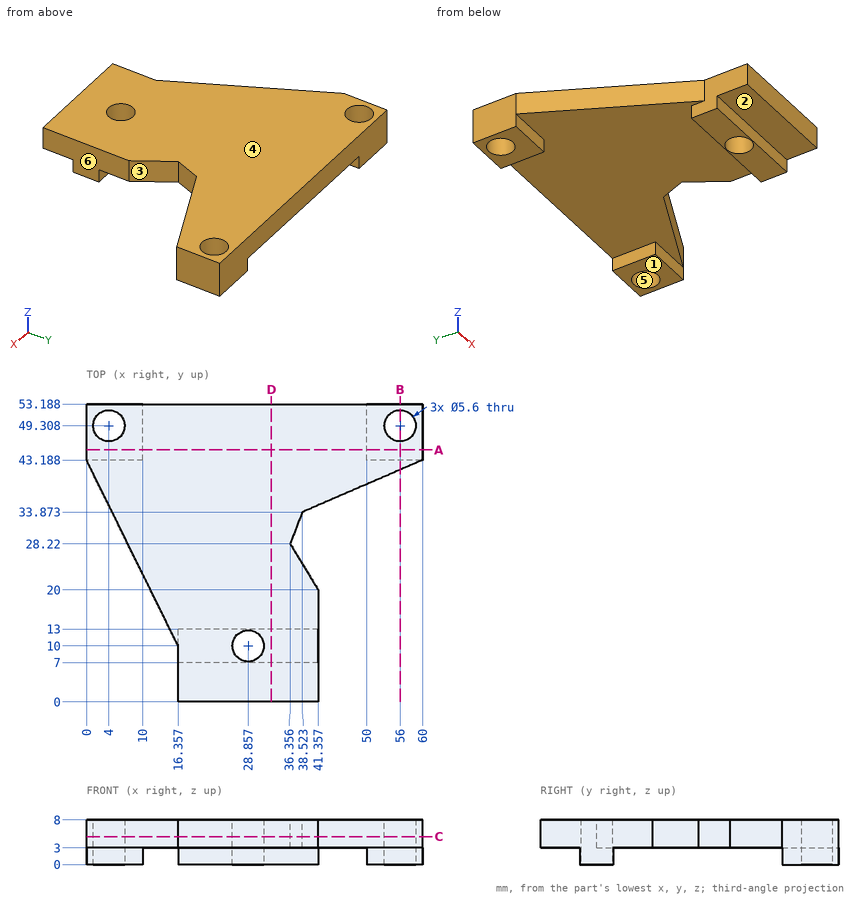
The drawing under review shows one solid part. Ordinate dimensions are in mm from its lowest x, y, z. A direction names the side the tool comes from. Give positions to 0.01 mm unless a question says otherwise; leave off trailing zeros. Order: outer loops, then holes, each group sorted by start corner. A loop starts at its lowest first (then second) coordinate and runs counter-clockwise, first axis right, second up. Notation, with made-up numbers: M 68.5,21.5 L 75.5,21.5 A18 cw 75.5,54.5 Z; hole C 31,-27.5 d10. An arc over 180 degrees is marked long. Answer in a Markdown table with one row per item. Add a question column.
1. Add section D-D on x = 33. State the section outline as (y, z) points, plus the area to 3 significant figures.
2. Mouldability with a two-part tool opening along X and no side actions: class the marked faces 4, 5 and 6 as released by +X, released by -X, zero draft, split by the parting line, or undercut.
3. Add section B-B on x = 56. State the section outline as (y, z) points.
4. Add section C-C on z = 5. State the section outline as (x, y) points (1 decimal).
5. To check wall thickness, follow line 1 along Y through (x, z) = (26.5, 6.5) (1 decimal); line 2 along Z through (x, y) = (26, 46); line 3 along X through (y, z) = (48.5, 5.5). State the ranges of each line that lie inside material, in increasing order.
6. Add section A-A on y = 45. State the section outline as (x, z) points.
7. Machinability: for the marked faces 1, 2 and 3, which of the approach directions +Z, -Z, +X, -X, +Y, -Y give a long, thin tool a straight path to every point of the face, cutting with its end or side? Answer none if there is none.
8. For pin 1 Ø6.5 at (x, y) = (4, 49.31) entering from +Z; pin 2 Ø0.9 at (x, z) = (2.5, 2) entering from -Y; pin 3 Ø1.5 at (x, z) = (27.5, 2) entering from +Y; pin 4 Ø1.5 at (x, z) = (33, 1.5) entering from -Y, all flat-tipped, find the tip position at first contact; note any pin that passes through.
The answers:
| question | item | result |
|---|---|---|
| 1 | outline | M 0,3 L 7,3 L 7,0 L 13,0 L 13,3 L 53.19,3 L 53.19,8 L 0,8 Z |
| 1 | area | 284 mm2 |
| 2 | face 4 | zero draft |
| 2 | face 5 | undercut |
| 2 | face 6 | released by +X |
| 3 | outline | M 41.45,3 L 43.19,3 L 43.19,0 L 46.51,0 L 46.51,8 L 41.45,8 Z; M 52.11,0 L 53.19,0 L 53.19,8 L 52.11,8 Z |
| 4 | outline | M 0,43.2 L 16.4,10 L 16.4,0 L 41.4,0 L 41.4,20 L 36.4,28.2 L 38.5,33.9 L 60,43.2 L 60,53.2 L 0,53.2 Z; hole C 4,49.3 d5.6; hole C 28.9,10 d5.6; hole C 56,49.3 d5.6 |
| 5 | line 1 | 0 to 8.5, 11.5 to 53.2 |
| 5 | line 2 | 3 to 8 |
| 5 | line 3 | 0 to 1.32, 6.68 to 53.32, 58.68 to 60 |
| 6 | outline | M 0,0 L 10,0 L 10,3 L 50,3 L 50,0 L 60,0 L 60,8 L 0,8 Z |
| 7 | face 1 | -Z, +X, -X, +Y, -Y |
| 7 | face 2 | -Z, +X, -X, -Y |
| 7 | face 3 | +Z, -Z, +X |
| 8 | pin 1 | z = 8 |
| 8 | pin 2 | y = 43.19 |
| 8 | pin 3 | y = 13 |
| 8 | pin 4 | y = 7 |
